from build123d import *

# Parameters (mm, degrees)
SCHIZZO2_R               = 3.75
TAGLIO_ESTRUSIONE1_DEPTH = 8
FILLET1_R                = 1


with BuildPart() as part:
    # Schizzo1 → Rivoluzione1 (revolve)
    with BuildSketch(Plane.XY):
        Polygon((0, 0), (12, 0), (12, 7), (7.5, 14), (0, 14), align=None)
    revolve(axis=Axis((0, -9.987677887, 0), (0, 1, 0)))

    # Schizzo2 → Taglio-Estrusione1 (cut)
    with BuildSketch(Plane(origin=(0, 14, 0), x_dir=(1, 0, 0), z_dir=(0, 1, 0))):
        Circle(SCHIZZO2_R)
    extrude(amount=-TAGLIO_ESTRUSIONE1_DEPTH, mode=Mode.SUBTRACT)

    # Fillet1
    fillet1_edges = [part.edges().sort_by_distance(p)[0] for p in [
        (-3.75, 14, 0),
        (-7.5, 14, 0),
        (-12, 7, 0),
    ]]
    fillet(fillet1_edges, radius=FILLET1_R)


solid = part.part
Verification items for the finished model (mm, model axes). A direction names the side the tool comes from. Give positions to 0.01 mm unless a question says otherwise; leave off trailing zeros. Order: outer loops, then holes, each group sorted by start corner. A loop starts at its lowest first (then second) coordinate and runs counter-clockwise, first axis right, second up. Notation, with made-up numbers: M 59,-19.5 L 102,-19.5 A15 cw 102,-15.5 Z; hole C 10.5,22 d2. An arc over 180 degrees is marked long. Answer as a JSON object with one key per item and string values. Group by question number.
1) Access from +Z, -Z, +X, -X, +Y, -Y to the whole of each face (thin tool, end or side, straight path). Record for faces 1 (the face through (1, 14, 5)), 2 (the face through (-3.746, 9.549, -0.165)).
2) Cross-section at A-A (y = 11.5). Enter the section's corners in (x, z).
3) Scan lines: line 1 along Z through (x, y) = (0, 11.5); line 2 along Z through (x, y) = (0, 11); line 3 along Y through (x, z) = (-4.5, 1.25). Record each from-to range of solid material in increasing order. Write a range as [from, to].
4) Depth check by flat-ended pin: pin 1 Ø1 at (y, z) = (9.5, 5.5) entering from -X; pin 2 Ø7 at (x, z) = (0, 0) entering from +Y; pin 3 Ø1.5 at (x, y) = (-5.5, 5) entering from +Z. Enter the tip coordinate at first touch or a pass-through.
5) Cross-section at B-B (y = 3.25). Enter the section's corners in (x, z), then the cut area to 3 significant figures.
6) Mould release check, pull along X, two halves, no side actions. Record for faces 3 (the face through (0, 0, 0)), 4 (the face through (0, 6, 0)), 5 (the face through (11.085, 3.4, 4.596)): released by +X, released by -X, zero draft, split by the parting line, or undercut.
Result sheet:
{
 "1": {"face 1": "+Z, -Z, +X, -X, +Y", "face 2": "+Y"},
 "2": {"outline": "C 0,0 d18.21; hole C 0,0 d7.5"},
 "3": {"line 1": "z = [-9.11, -3.75], [3.75, 9.11]", "line 2": "z = [-9.43, -3.75], [3.75, 9.43]", "line 3": "y = [0, 14]"},
 "4": {"pin 1": "stops at x = -9.29", "pin 2": "stops at y = 6", "pin 3": "stops at z = 11.02"},
 "5": {"outline": "C 0,0 d24", "area": "452 mm2"},
 "6": {"face 3": "zero draft", "face 4": "undercut", "face 5": "split by the parting line"}
}
